Input: part model. Units: mm. Frame: model coordinates. A direction names the side the tool comes from. Give positions to 0.01 mm unless a question says otherwise; leave off trailing zeros. Write each loop counter-clockwise with the first axis right and the second up, starting at its lowest first coordinate (ties: lowest second). Pieces come first, ordered by that corner, then holes. Notation, with made-up numbers: (2, -34.75) -> (37, -34.75) arc R11 ccw to (37, -24.75) -> close; hole circle Ø4 at (20.5, 70). An arc over 180 degrees is marked (long way). Answer as a JSON object with one key per item and string values. Group by question number.
from build123d import *

# Parameters (mm, degrees)
BOX001_W               = 50
BOX001_H               = 15
BOX001_DEPTH           = 4.8
CYLINDER006_R          = 7.4
CYLINDER006_DEPTH      = 10
BOX002_W               = 15
BOX002_H               = 21.5
BOX002_DEPTH           = 4.8
CYLINDER005_R          = 7.4
CYLINDER005_DEPTH      = 10
CYLINDER002_W          = 23
CYLINDER002_H          = 4.8
CYLINDER002_ANGLE      = 30
CYLINDER001_W          = 27
CYLINDER001_H          = 4.8
CYLINDER001_ANGLE      = 30
CUT001_PLACEMENT_ANGLE = 105
CYLINDER010_R          = 1.65
CYLINDER010_DEPTH      = 10
CYLINDER012_R          = 1.65
CYLINDER012_DEPTH      = 10
CYLINDER013_R          = 21
CYLINDER013_DEPTH      = 4.8
CYLINDER004_W          = 23
CYLINDER004_H          = 4.8
CYLINDER004_ANGLE      = 30
CYLINDER003_W          = 27
CYLINDER003_H          = 4.8
CYLINDER003_ANGLE      = 30
CUT002_PLACEMENT_ANGLE = 75
CYLINDER_R             = 30.1
CYLINDER_DEPTH         = 10
BOX_W                  = 70
BOX_H                  = 70
BOX_DEPTH              = 14.8


with BuildPart() as obj1:
    # Box001 → Box001 (new body)
    with BuildSketch(Plane(origin=(-25, -7.5, 0), x_dir=(1, 0, 0), z_dir=(0, 0, 1))):
        with Locations((25, 7.5)):
            Rectangle(BOX001_W, BOX001_H)
    extrude(amount=BOX001_DEPTH)


with BuildPart() as cylinder006:
    # Cylinder006 → Cylinder006 (new body)
    with BuildSketch(Plane(origin=(35, 0, 7.4), x_dir=(0, 0, -1), z_dir=(1, 0, 0))):
        Circle(CYLINDER006_R)
    extrude(amount=CYLINDER006_DEPTH)


with BuildPart() as obj2:
    # Box002 → Box002 (new body)
    with BuildSketch(Plane(origin=(-7.5, -21.5, 0), x_dir=(1, 0, 0), z_dir=(0, 0, 1))):
        with Locations((7.5, 10.75)):
            Rectangle(BOX002_W, BOX002_H)
    extrude(amount=BOX002_DEPTH)


with BuildPart() as fusion001:
    # Cylinder005 → Cylinder005 (new body)
    with BuildSketch(Plane(origin=(-45, 0, 7.4), x_dir=(0, 0, -1), z_dir=(1, 0, 0))):
        Circle(CYLINDER005_R)
    extrude(amount=CYLINDER005_DEPTH)

    # Fusion001: union obj1, Cylinder006, obj2
    add(obj1.part)
    add(cylinder006.part)
    add(obj2.part)


with BuildPart() as zylinder002:
    # Cylinder002 → Cylinder002 (revolve)
    with BuildSketch(Plane.XZ):
        with Locations((11.5, 2.4)):
            Rectangle(CYLINDER002_W, CYLINDER002_H)
    revolve(axis=Axis((0, 0, 0), (0, 0, 1)), revolution_arc=CYLINDER002_ANGLE)


with BuildPart() as cut004:
    # Cylinder001 → Cylinder001 (revolve)
    with BuildSketch(Plane.XZ):
        with Locations((13.5, 2.4)):
            Rectangle(CYLINDER001_W, CYLINDER001_H)
    revolve(axis=Axis((0, 0, 0), (0, 0, 1)), revolution_arc=CYLINDER001_ANGLE)

    # Cut001: cut Zylinder002
    add(zylinder002.part, mode=Mode.SUBTRACT)


with BuildPart() as cut004_1:
    # Cut001 placement: moved
    add(cut004.part.rotate(Axis((0, 0, 0), (0, 0, -1)), CUT001_PLACEMENT_ANGLE))


with BuildPart() as cylinder010:
    # Cylinder010 → Cylinder010 (new body)
    with BuildSketch(Plane(origin=(-35, -30, 7.5), x_dir=(0, 0, -1), z_dir=(1, 0, 0))):
        Circle(CYLINDER010_R)
    extrude(amount=CYLINDER010_DEPTH)


with BuildPart() as cylinder012:
    # Cylinder012 → Cylinder012 (new body)
    with BuildSketch(Plane(origin=(25, -30, 7.5), x_dir=(0, 0, -1), z_dir=(1, 0, 0))):
        Circle(CYLINDER012_R)
    extrude(amount=CYLINDER012_DEPTH)


with BuildPart() as cylinder013:
    # Cylinder013 → Cylinder013 (new body)
    with BuildSketch(Plane.XY):
        Circle(CYLINDER013_R)
    extrude(amount=CYLINDER013_DEPTH)


with BuildPart() as zylinder004:
    # Cylinder004 → Cylinder004 (revolve)
    with BuildSketch(Plane.XZ):
        with Locations((11.5, 2.4)):
            Rectangle(CYLINDER004_W, CYLINDER004_H)
    revolve(axis=Axis((0, 0, 0), (0, 0, 1)), revolution_arc=CYLINDER004_ANGLE)


with BuildPart() as obj3:
    # Cylinder003 → Cylinder003 (revolve)
    with BuildSketch(Plane.XZ):
        with Locations((13.5, 2.4)):
            Rectangle(CYLINDER003_W, CYLINDER003_H)
    revolve(axis=Axis((0, 0, 0), (0, 0, 1)), revolution_arc=CYLINDER003_ANGLE)

    # Cut002: cut Zylinder004
    add(zylinder004.part, mode=Mode.SUBTRACT)


with BuildPart() as obj3_1:
    # Cut002 placement: moved
    add(obj3.part.rotate(Axis((0, 0, 0), (0, 0, 1)), CUT002_PLACEMENT_ANGLE))

    # Fusion: union Cut004, Cylinder010, Cylinder012, Cylinder013
    add(cut004_1.part)
    add(cylinder010.part)
    add(cylinder012.part)
    add(cylinder013.part)


with BuildPart() as zylinder:
    # Cylinder → Cylinder (new body)
    with BuildSketch(Plane.XY.offset(4.8)):
        Circle(CYLINDER_R)
    extrude(amount=CYLINDER_DEPTH)


with BuildPart() as fusion002:
    # Box → Box (new body)
    with BuildSketch(Plane(origin=(-35, -35, 0), x_dir=(1, 0, 0), z_dir=(0, 0, 1))):
        with Locations((35, 35)):
            Rectangle(BOX_W, BOX_H)
    extrude(amount=BOX_DEPTH)

    # Cut: cut Zylinder
    add(zylinder.part, mode=Mode.SUBTRACT)

    # Cut003: cut obj3
    add(obj3_1.part, mode=Mode.SUBTRACT)

    # Fusion002: union Fusion001
    add(fusion001.part)


solid = fusion002.part
1. Section D-D (x = -3.5). Return the cut outline in (y, z).
2. Reachability of faces 1 (the face through (-6.525, -29.384, 9.73)), 2 (the face through (6.463, 24.121, 2.434)), 3 (the face through (25, -30, 8)) from +Z, -Z, +X, -X, +Y, -Y: full face, straight path, thin tool, end or side. Return the list, or none.
3. Contact query for flat-ended pins moving along their axis: pin 1 Ø1 at (y, z) = (-30.5, 7) entering from -X; pin 2 Ø1.5 at (y, z) = (25.5, 4.5) entering from -X; pin 3 Ø4 at (x, y) = (2, -25.5) entering from +Z. Output: stop coordinate, or through.
4. Line query: line 1 (X direction, y = -1, z = 8); line 2 (Y direction, x = 2.5, z = 3.5); line 3 (Y direction, x = 0, z = 10.25). Output: solid intervals per line, ascending.
5. Section C-C (y = 16). Return the cut outline in (x, z).
6. Section A-A (x = 14). Return the cut outline in (y, z).
7. Mould query, pull axis X, two halves, no side actions, for faces 4 (the face through (45, 0, 8)), 5 (the face through (0, -35, 7)), 6 (the face through (0, 0, 4.8)). Classes: pulls with the +X half, pulls with the -X half, needs draft (parallel to the pull), parting line crosses it, or undercut.
8. Section B-B (z = 11). Return the cut outline in (x, y), plus the area to 3 significant figures.
Working result:
{
 "1": {"outline": "(-35, 0) -> (-26.77, 0) -> (-26.77, 4.8) -> (-29.9, 4.8) -> (-29.9, 14.8) -> (-35, 14.8) -> close; (-22.73, 0) -> (7.5, 0) -> (7.5, 4.8) -> (-22.73, 4.8) -> close; (20.71, 0) -> (22.73, 0) -> (22.73, 4.8) -> (20.71, 4.8) -> close; (26.77, 0) -> (35, 0) -> (35, 14.8) -> (29.9, 14.8) -> (29.9, 4.8) -> (26.77, 4.8) -> close"},
 "2": {"face 1": "+Z", "face 2": "+Z, -Z", "face 3": "+X"},
 "3": {"pin 1": "stops at x = -25", "pin 2": "stops at x = -35", "pin 3": "stops at z = 4.8"},
 "4": {"line 1": "x = -45 to -30.08, 30.08 to 45", "line 2": "y = -35 to -26.88, -22.86 to 7.5, 20.85 to 22.86, 26.88 to 35", "line 3": "y = -35 to -30.1, 30.1 to 35"},
 "5": {"outline": "(-35, 0) -> (-13.6, 0) -> (-13.6, 4.8) -> (-25.5, 4.8) -> (-25.5, 14.8) -> (-35, 14.8) -> close; (13.6, 0) -> (35, 0) -> (35, 14.8) -> (25.5, 14.8) -> (25.5, 4.8) -> (13.6, 4.8) -> close"},
 "6": {"outline": "(-35, 0) -> (-15.65, 0) -> (-15.65, 4.8) -> (-26.65, 4.8) -> (-26.65, 14.8) -> (-35, 14.8) -> close; (-7.5, 0) -> (7.5, 0) -> (7.5, 4.8) -> (-7.5, 4.8) -> close; (15.65, 0) -> (35, 0) -> (35, 14.8) -> (26.65, 14.8) -> (26.65, 4.8) -> (15.65, 4.8) -> close"},
 "7": {"face 4": "pulls with the +X half", "face 5": "needs draft", "face 6": "undercut"},
 "8": {"outline": "(-45, -6.47) -> (-35, -6.47) -> (-35, -35) -> (35, -35) -> (35, -6.47) -> (45, -6.47) -> (45, 6.47) -> (35, 6.47) -> (35, 35) -> (-35, 35) -> (-35, 6.47) -> (-45, 6.47) -> close; hole circle Ø60.2 at (0, 0)", "area": "2,310 mm^2"}
}
